```python
from build123d import *

# Parameters (mm, degrees)
ESQUISSE2_R             = 2.98
BOSS_EXTRU_1_DEPTH      = 7.9
BOSS_EXTRU_2_DEPTH      = 0.5
BOSS_EXTRU_2_DEPTH_BACK = 0.5
ESQUISSE3_W             = 40.6
ESQUISSE3_H             = 35.8
CHANFREIN1_SIZE         = 1


with BuildPart() as part:
    # Esquisse2 → Boss.-Extru.1 (new body)
    with BuildSketch(Plane(origin=(0, 0, 0), x_dir=(1, 0, 0), z_dir=(0, 1, 0))):
        with Locations(Location((0, 0, 0), (0, 0, 270))):
            Circle(ESQUISSE2_R)
    extrude(amount=-BOSS_EXTRU_1_DEPTH)

    # Esquisse3 → Boss.-Extru.2 (add, two sides: drawn at the far end of the back side and taken through both)
    with BuildSketch(Plane.XY.offset(-BOSS_EXTRU_2_DEPTH_BACK)):
        with Locations((0, 17.9)):
            Rectangle(ESQUISSE3_W, ESQUISSE3_H)
    extrude(amount=BOSS_EXTRU_2_DEPTH + BOSS_EXTRU_2_DEPTH_BACK)

    # Chanfrein1
    chanfrein1_edges = [part.edges().sort_by_distance(p)[0] for p in [
        (-20.3, 35.8, 0),
        (20.3, 35.8, 0),
    ]]
    chamfer(chanfrein1_edges, length=CHANFREIN1_SIZE)


solid = part.part
```
Could you check a few things on this model? Use its own coordinates, in mm. A direction names the side the tool comes from. Round coordinates to 2 decimals unless told otherwise and drop trailing zeros. Write each loop counter-clockwise with the first axis right and the second up, starting at its lowest first coordinate (ties: lowest second). Pieces come first, ordered by that corner, then holes. Notation, with made-up numbers: M 38,-28.5 L 49,-28.5 A16 ccw 49,-21.5 Z; hole C 30.5,41.25 d9. An arc over 180 degrees is marked long. Answer in a Markdown table with one row per item. Add a question column.
Q1. On a 3-axis mill with a long thin cutter (end or side, diameter ignored), from which of +Z, -Z, +X, -X, +Y, -Y can I reach the whole of each face in a straight line? I mean faces 1 (the flat face through (11, 0, 0)), 2 (the flat face through (-12, 0, 0)), 3 (the flat face through (-19.8, 35.3, 0)), 4 (the flat face through (0, 0, -1)), 5 (the flat face through (0, 0, 1)). Say none if no direction works.
Q2. Will these pins go through, and if not, where does the flat tip stop? pin 1 Ø8 at (x, y) = (5, 0) entering from +Z; pin 2 Ø5 at (x, y) = (5, 10) entering from -Z; pin 3 Ø1.2 at (x, z) = (0, 2) entering from +Y.
Q3. If I drill on line 1 (Z direction, x = -19, y = 33.5); line 2 (Y direction, x = 18, z = -0.3); line 3 (X direction, y = -2, z = -2.4), over which ranges is the centre line in solid material (lowest first)? Write a range as from..to.
Q4. Imagine slicing it at A-A (z = 0). Please give me the cut outline in (x, y).
Q5. Imagine slicing it at B-B (x = 0). Please give me the cut outline in (y, z), then the cut area to 3 significant figures.
Q6. Imagine slicing it at D-D (z = -2.45). Please give me the cut outline in (x, y), then the cut area to 3 significant figures.
Q7. Imagine slicing it at C-C (y = 24.5). Please give me the cut outline in (x, z), then the cut area to 3 significant figures.
Values:
| question | item | result |
|---|---|---|
| 1 | face 1 | +Z, -Z, +X, -Y |
| 1 | face 2 | +Z, -Z, -X, -Y |
| 1 | face 3 | +Z, -Z, -X, +Y |
| 1 | face 4 | -Z, +X, -X, +Y |
| 1 | face 5 | +Z, +X, -X, +Y |
| 2 | pin 1 | z = 2.81 |
| 2 | pin 2 | z = -0.5 |
| 2 | pin 3 | y = 0 |
| 3 | line 1 | -0.5..0.5 |
| 3 | line 2 | 0..35.8 |
| 3 | line 3 | -1.77..1.77 |
| 4 | outline | M -20.3,0 L -2.98,0 L -2.98,-7.9 L 2.98,-7.9 L 2.98,0 L 20.3,0 L 20.3,34.8 L 19.3,35.8 L -19.3,35.8 L -20.3,34.8 Z |
| 5 | outline | M -7.9,-2.98 L 0,-2.98 L 0,-0.5 L 35.8,-0.5 L 35.8,0.5 L 0,0.5 L 0,2.98 L -7.9,2.98 Z |
| 5 | area | 82.9 mm^2 |
| 6 | outline | M -1.7,-7.9 L 1.7,-7.9 L 1.7,0 L -1.7,0 Z |
| 6 | area | 26.8 mm^2 |
| 7 | outline | M -20.3,-0.5 L 20.3,-0.5 L 20.3,0.5 L -20.3,0.5 Z |
| 7 | area | 40.6 mm^2 |
